Can you work these out from the drawing? Everything is in mm from the part's minimum corner. A direction names the side the tool comes from. Round coordinates to 2 decimals unless told otherwise and drop trailing zeros. Write each loop counter-clockwise with the first axis right and the second up, starting at its lowest first coordinate (ties: lowest second). Pieces come first, ordered by that corner, then holes. Notation, with made-up numbers: (70, 62) - (116, 62) arc R24 ccw to (116, 99) - close; hole circle Ø3 at (-20, 39.25). An arc over 180 degrees is marked (long way). One line per item, written item: value. Start each with the question number.
(1) I want a section at C-C on x = 15. List the corners of the cut face in (y, z) for me.
(2) I want a section at B-B on z = 0.5. List the corners of the cut face in (x, y) for me.
(3) I'm going to push flat-ended pins straight in: pin 1 Ø1.5 at (x, z) = (8, 1) entering from +Y; pin 2 Ø1 at (x, z) = (31, 1) entering from +Y. Where does each tip first touch, or does it pass through?
(4) If I drill on L1, parallel to Y at x = 28, z = 0.75; L2, parallel to X at y = 8.5, z = 2.7; L3, parallel to Y at x = 14, z = 1.9, over which ranges is the centre line in solid material (lowest first)? Write a range as from..to.
(5) Thinking about a two-plate mould opening in Y: for the marked faces 1, 2, 3 and 4, which applies, +Y half, -Y half, draft (parallel to the pull), parting line (faces both ways), or undercut?
(6) I want a section at D-D on y = 17. List the corners of the cut face in (x, z) for me.
(7) I want a section at A-A on x = 28. List the corners of the cut face in (y, z) for me.
(8) On a 3-axis mill with a long thin cutter (end or side, diameter ignored), from which of +Z, -Z, +X, -X, +Y, -Y can I reach the whole of each face in a straight line? I mean the marked faces 5 and 6. Say none if no direction works.
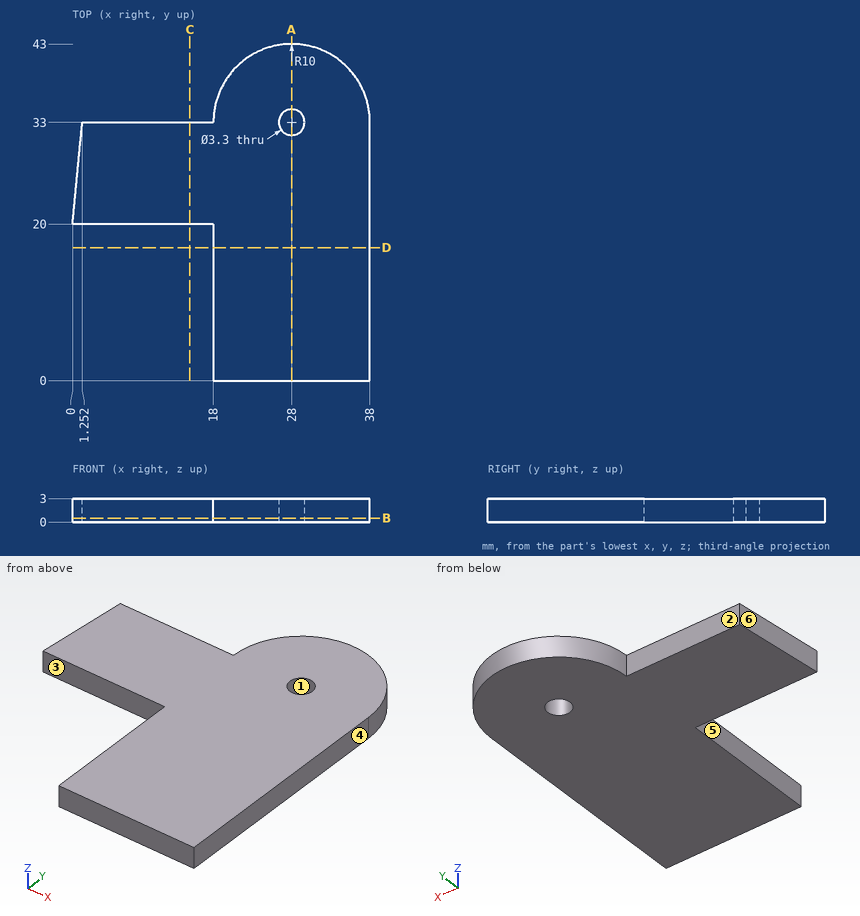
Established:
1. outline: (20, 0) - (33, 0) - (33, 3) - (20, 3) - close
2. outline: (0, 20) - (18, 20) - (18, 0) - (38, 0) - (38, 33) arc R10 ccw to (18, 33) - (1.25, 33) - close; hole circle Ø3.3 at (28, 33)
3. pin 1: y = 33
3. pin 2: y = 42.68
4. L1: 0..31.35, 34.65..43
4. L2: 18..38
4. L3: 20..33
5. face 1: undercut
5. face 2: +Y half
5. face 3: -Y half
5. face 4: draft
6. outline: (18, 0) - (38, 0) - (38, 3) - (18, 3) - close
7. outline: (0, 0) - (31.35, 0) - (31.35, 3) - (0, 3) - close; (34.65, 0) - (43, 0) - (43, 3) - (34.65, 3) - close
8. face 5: +Z, -Z, -X, -Y
8. face 6: +Z, -Z, -X, +Y
